```python
from build123d import *

# Parameters (mm, degrees)
CYLINDER010_R     = 1.55
CYLINDER010_DEPTH = 10
CYLINDER_R        = 1
CYLINDER_DEPTH    = 10
CYLINDER009_R     = 1.55
CYLINDER009_DEPTH = 10
CYLINDER011_R     = 3
CYLINDER011_DEPTH = 1.7
BOX_W             = 5
BOX_H             = 19
BOX_DEPTH         = 1.7
FILLET_R          = 1
CYLINDER012_R     = 3
CYLINDER012_DEPTH = 1.7


with BuildPart() as threadedhole006:
    # Cylinder010 → Cylinder010 (new body)
    with BuildSketch(Plane(origin=(0, 8, 0), x_dir=(1, 0, 0), z_dir=(0, 0, 1))):
        Circle(CYLINDER010_R)
    extrude(amount=CYLINDER010_DEPTH)


with BuildPart() as cylinder:
    # Cylinder → Cylinder (new body)
    with BuildSketch(Plane.XY):
        Circle(CYLINDER_R)
    extrude(amount=CYLINDER_DEPTH)


with BuildPart() as fusion005:
    # Cylinder009 → Cylinder009 (new body)
    with BuildSketch(Plane(origin=(0, -7, 0), x_dir=(1, 0, 0), z_dir=(0, 0, 1))):
        Circle(CYLINDER009_R)
    extrude(amount=CYLINDER009_DEPTH)

    # Fusion005: union ThreadedHole006, Cylinder
    add(threadedhole006.part)
    add(cylinder.part)


with BuildPart() as threadedhole007:
    # Cylinder011 → Cylinder011 (new body)
    with BuildSketch(Plane(origin=(0, 8, 0), x_dir=(1, 0, 0), z_dir=(0, 0, 1))):
        Circle(CYLINDER011_R)
    extrude(amount=CYLINDER011_DEPTH)


with BuildPart() as fillet_body:
    # Box → Box (new body)
    with BuildSketch(Plane(origin=(-2.5, -9, 0), x_dir=(1, 0, 0), z_dir=(0, 0, 1))):
        with Locations((2.5, 9.5)):
            Rectangle(BOX_W, BOX_H)
    extrude(amount=BOX_DEPTH)

    # Fillet
    fillet_edges = [fillet_body.edges().sort_by_distance(p)[0] for p in [
        (-2.5, -9, 0.85),
        (-2.5, 10, 0.85),
        (2.5, -9, 0.85),
        (2.5, 10, 0.85),
    ]]
    fillet(fillet_edges, radius=FILLET_R)


with BuildPart() as cut:
    # Cylinder012 → Cylinder012 (new body)
    with BuildSketch(Plane(origin=(0, -7, 0), x_dir=(1, 0, 0), z_dir=(0, 0, 1))):
        Circle(CYLINDER012_R)
    extrude(amount=CYLINDER012_DEPTH)

    # Fusion: union ThreadedHole007, Fillet body
    add(threadedhole007.part)
    add(fillet_body.part)

    # Cut: cut Fusion005
    add(fusion005.part, mode=Mode.SUBTRACT)


solid = cut.part
```
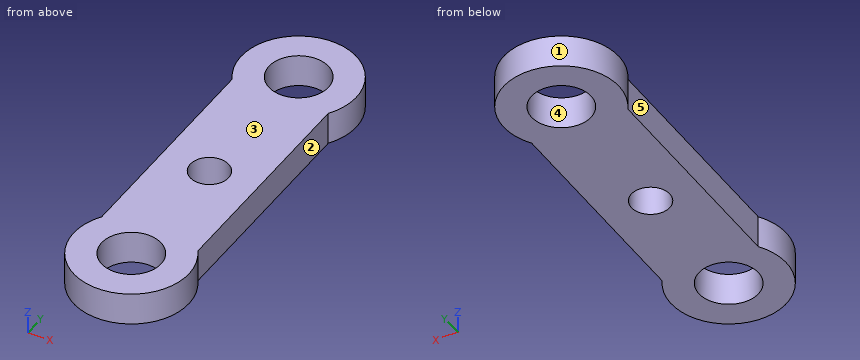
Check sheet for the modelled part. Datum: model origin and axes. Units: mm. Face numbers are marked on the shaded views. A direction names the side the tool comes from. Coordinates: 2 decimals unless noted, no trailing zeros. Order: outer loops, then holes, each group sorted by start corner. A loop starts at its lowest first (then second) coordinate and runs counter-clockwise, first axis right, second up. Notation, with made-up numbers: M -3,57.25 L 16,57.25 A26 ccw 16,90.25 Z; hole C 79,27 d6. An arc over 180 degrees is marked long. Write each question's results on one line, items separated by ' | '. Start each with the question number.
1. Go/stop test with flat-tipped pins: P1, Ø0.8, axis at y = 1.5, z = 0.5, coming from the -X side; P2, Ø1, axis at x = 1.5, z = 0.5, coming from the -Y side; P3, Ø0.5, axis at y = -1, z = 0.5, coming from the +X side. Record where each tip stops, or that it passes through.
2. Access from +Z, -Z, +X, -X, +Y, -Y to the whole of each face (thin tool, end or side, straight path). Record for the marked faces 1 and 2.
3. Cross-section at C-C on z = 1.4. Record the cut outline in (x, y).
4. Cross-section at D-D on y = -7. Record the cut outline in (x, z).
5. Cross-section at A-A on y = 0. Record the cut outline in (x, z).
6. Material ranges on probe 1 along X at (y, z) = (0, 0.5); probe 2 along Y at (x, z) = (1.3, 0.55); probe 3 along X at (y, z) = (-7, 1.2), recorded low to high.
7. Mould release check, pull along X, two halves, no side actions. Record for the marked faces 3, 4 and 5: +X half, -X half, draft (parallel to the pull), parting line (faces both ways), or undercut.
8. Cross-section at B-B on x = 0. Record the cut outline in (y, z).
Checks:
1) P1: stops at x = -2.5 | P2: stops at y = -9.83 | P3: stops at x = 2.5
2) face 1: +Z, -Z | face 2: +Z, -Z, +X
3) outline: M -2.5,-5.34 A3 ccw long 2.5,-5.34 L 2.5,6.34 A3 ccw long -2.5,6.34 Z; hole C 0,-7 d3.1; hole C 0,8 d3.1; hole C 0,0 d2
4) outline: M -3,0 L -1.55,0 L -1.55,1.7 L -3,1.7 Z; M 1.55,0 L 3,0 L 3,1.7 L 1.55,1.7 Z
5) outline: M -2.5,0 L -1,0 L -1,1.7 L -2.5,1.7 Z; M 1,0 L 2.5,0 L 2.5,1.7 L 1,1.7 Z
6) probe 1: x = -2.5 to -1, 1 to 2.5 | probe 2: y = -9.7 to -7.84, -6.16 to 7.16, 8.84 to 10.7 | probe 3: x = -3 to -1.55, 1.55 to 3
7) face 3: draft | face 4: undercut | face 5: -X half
8) outline: M -10,0 L -8.55,0 L -8.55,1.7 L -10,1.7 Z; M -5.45,0 L -1,0 L -1,1.7 L -5.45,1.7 Z; M 1,0 L 6.45,0 L 6.45,1.7 L 1,1.7 Z; M 9.55,0 L 11,0 L 11,1.7 L 9.55,1.7 Z
